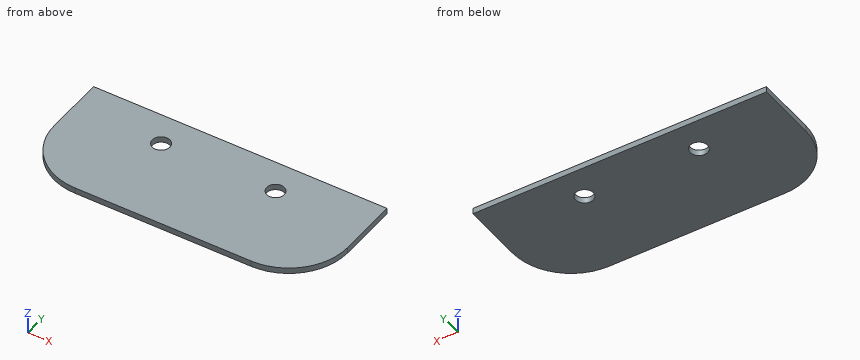
from build123d import *

# Parameters (mm, degrees)
SKETCH1_W           = 50
SKETCH1_H           = 20.400620127
SKETCH1_R           = 1.5
BOSS_EXTRUDE1_DEPTH = 1
FILLET3_R           = 10
FILLET5_R           = 10


with BuildPart() as part:
    # Sketch1 → Boss-Extrude1 (new body)
    with BuildSketch(Plane.XY):
        with Locations((25, 10.200310063)):
            Rectangle(SKETCH1_W, SKETCH1_H)
        with Locations((15, 15)):
            Circle(SKETCH1_R, mode=Mode.SUBTRACT)
        with Locations((34.5, 15)):
            Circle(SKETCH1_R, mode=Mode.SUBTRACT)
    extrude(amount=BOSS_EXTRUDE1_DEPTH)

    # Fillet3
    fillet3_edges = [part.edges().sort_by_distance(p)[0] for p in [
        (0, 0, 0.5),
    ]]
    fillet(fillet3_edges, radius=FILLET3_R)

    # Fillet5
    fillet5_edges = [part.edges().sort_by_distance(p)[0] for p in [
        (50, 0, 0.5),
    ]]
    fillet(fillet5_edges, radius=FILLET5_R)


solid = part.part
Can you work these out from the model? Positions are in its coordinate system, mm. Round coordinates to 2 decimals unless told otherwise and drop trailing zeros. Loops run counter-clockwise (first coordinate to the right, second up) from the corner with the lowest first, then second, coordinate; pieces in that order, holes last. Notation, with made-up numbers: (64, 40.5) - (118, 40.5) arc R16 ccw to (118, 45.5) - close; hole circle Ø3 at (-6, 80). An arc over 180 degrees is marked (long way). Use CSV: the item, a comma, the result in double quotes. Start each with the question number.
1) For pin 1 Ø3 at (x, y) = (31.5, 15) entering from -Z; pin 2 Ø1.8 at (x, y) = (34.5, 15) entering from +Z, each with a flat end and sliding along its axis, tell me the tip position at first contact or that it passes through.
2) If we section it at B-B on y = 15: Write out the boundary of the cut face in (x, z), plus the area to 3 significant figures.
3) If we section it at D-D on x = 43.5: Write out the boundary of the cut face in (y, z).
4) Please list where these lines run through material, in increasing order: probe 1 along Y at (x, z) = (34.5, 0.3); probe 2 along Y at (x, z) = (34, 0.2); probe 3 along X at (y, z) = (5, 0.15). Write a range as [from, to].
5) If we section it at C-C on z = 0.6: Write out the boundary of the cut face in (x, y), plus the area to 3 significant figures.
6) If we section it at A-A on x = 34.5: Write out the boundary of the cut face in (y, z), plus the area to 3 significant figures.
Geometry results:
1,pin 1,"stops at z = 0"
1,pin 2,"passes through"
2,outline,"(0, 0) - (13.5, 0) - (13.5, 1) - (0, 1) - close; (16.5, 0) - (33, 0) - (33, 1) - (16.5, 1) - close; (36, 0) - (50, 0) - (50, 1) - (36, 1) - close"
2,area,"44.0 mm2"
3,outline,"(0.63, 0) - (20.4, 0) - (20.4, 1) - (0.63, 1) - close"
4,probe 1,"y = [0, 13.5], [16.5, 20.4]"
4,probe 2,"y = [0, 13.59], [16.41, 20.4]"
4,probe 3,"x = [1.34, 48.66]"
5,outline,"(0, 10) arc R10 ccw to (10, 0) - (40, 0) arc R10 ccw to (50, 10) - (50, 20.4) - (0, 20.4) - close; hole circle Ø3 at (15, 15); hole circle Ø3 at (34.5, 15)"
5,area,"963 mm2"
6,outline,"(0, 0) - (13.5, 0) - (13.5, 1) - (0, 1) - close; (16.5, 0) - (20.4, 0) - (20.4, 1) - (16.5, 1) - close"
6,area,"17.4 mm2"
